```python
from build123d import *
from OCP.BRepFilletAPI import BRepFilletAPI_MakeChamfer

# Parameters (mm, degrees)
BOSS_EXTRUDE1_DEPTH                               = 38
SKETCH5_W                                         = 63
SKETCH5_H                                         = 38
BOSS_EXTRUDE2_DEPTH                               = 1.6
CHAMFER6_SIZE                                     = 0.8
CHAMFER6_SIZE2                                    = 0.738449877
CHAMFER7_SIZE                                     = 0.8
CHAMFER7_SIZE2                                    = 0.880050294
CHAMFER7_SIZE2_2                                  = 0.59857957
CSK_FOR_6_FLAT_HEAD_MACHINE_SCREW_100_D           = 4.3053
CSK_FOR_6_FLAT_HEAD_MACHINE_SCREW_100_DEPTH       = 3.6
CSK_FOR_6_FLAT_HEAD_MACHINE_SCREW_100_CSINK_D     = 7.0866
CSK_FOR_6_FLAT_HEAD_MACHINE_SCREW_100_CSINK_ANGLE = 100
FILLET1_R                                         = 10
CHAMFER10_SIZE                                    = 1.5


with BuildPart() as part:
    # Sketch1 → Boss-Extrude1 (new body)
    with BuildSketch(Plane.XY):
        Polygon((-34.595581798, 39), (-29.986555798, 39), (-32.97810591, 45.15618727), (-31.179250624, 46.030326652), (-27.76291945, 39), (-27.76291945, 37), (-32.76291945, 37), (-36, 0), (0, 0), (36, 0), (32.76291945, 37), (27.76291945, 37), (27.76291945, 39), (31.179250624, 46.030326652), (32.97810591, 45.15618727), (29.986555798, 39), (34.595581798, 39), (38.182617002, -2), (0, -2), (-38.182617002, -2), align=None)
    extrude(amount=BOSS_EXTRUDE1_DEPTH)

    # Sketch5 → Boss-Extrude2 (add)
    with BuildSketch(Plane.XZ.offset(2)):
        with Locations((0, 19)):
            Rectangle(SKETCH5_W, SKETCH5_H)
    extrude(amount=BOSS_EXTRUDE2_DEPTH)

    # Chamfer6: one chamfer whose edges measure the first distance from different faces: ONE call of the kernel's chamfer builder (chamfer() names one face for all edges)
    chamfer6_edges_1 = [part.edges().sort_by_distance(p)[0] for p in [
        (-36, 0, 19),
    ]]
    chamfer6_side_1 = [part.faces().sort_by_distance(p)[0] for p in [
        (0, 0, 19),
    ]]
    chamfer6_edges_2 = [part.edges().sort_by_distance(p)[0] for p in [
        (36, 0, 19),
    ]]
    chamfer6_side_2 = [part.faces().sort_by_distance(p)[0] for p in [
        (34.381459725, 18.5, 19),
    ]]
    chamfer6_edges_3 = [part.edges().sort_by_distance(p)[0] for p in [
        (38.182617002, -2, 19),
    ]]
    chamfer6_side_3 = [part.faces().sort_by_distance(p)[0] for p in [
        (34.841308501, -2, 19),
    ]]
    chamfer6_edges_4 = [part.edges().sort_by_distance(p)[0] for p in [
        (-38.182617002, -2, 19),
    ]]
    chamfer6_side_4 = [part.faces().sort_by_distance(p)[0] for p in [
        (-36.3890994, 18.5, 19),
    ]]
    chamfer6 = BRepFilletAPI_MakeChamfer(part.part.solid().wrapped)
    for e in chamfer6_edges_1:
        chamfer6.Add(CHAMFER6_SIZE, CHAMFER6_SIZE2, e.wrapped, chamfer6_side_1[0].wrapped)  # the first distance lies on this face
    for e in chamfer6_edges_2:
        chamfer6.Add(CHAMFER6_SIZE, CHAMFER6_SIZE2, e.wrapped, chamfer6_side_2[0].wrapped)  # the first distance lies on this face
    for e in chamfer6_edges_3:
        chamfer6.Add(CHAMFER6_SIZE, CHAMFER6_SIZE2, e.wrapped, chamfer6_side_3[0].wrapped)  # the first distance lies on this face
    for e in chamfer6_edges_4:
        chamfer6.Add(CHAMFER6_SIZE, CHAMFER6_SIZE2, e.wrapped, chamfer6_side_4[0].wrapped)  # the first distance lies on this face
    add(Compound.cast(chamfer6.Shape()), mode=Mode.REPLACE)

    # Chamfer7: one chamfer whose edges measure the first distance from different faces: ONE call of the kernel's chamfer builder (chamfer() names one face for all edges)
    chamfer7_edges_1 = [part.edges().sort_by_distance(p)[0] for p in [
        (-32.76291945, 37, 19),
    ]]
    chamfer7_side_1 = [part.faces().sort_by_distance(p)[0] for p in [
        (-34.349279651, 18.867819926, 19),
    ]]
    chamfer7_edges_2 = [part.edges().sort_by_distance(p)[0] for p in [
        (32.76291945, 37, 19),
    ]]
    chamfer7_side_2 = [part.faces().sort_by_distance(p)[0] for p in [
        (30.26291945, 37, 19),
    ]]
    chamfer7_edges_3 = [part.edges().sort_by_distance(p)[0] for p in [
        (29.986555798, 39, 19),
    ]]
    chamfer7_side_3 = [part.faces().sort_by_distance(p)[0] for p in [
        (32.291068798, 39, 19),
    ]]
    chamfer7_edges_4 = [part.edges().sort_by_distance(p)[0] for p in [
        (34.595581798, 39, 19),
    ]]
    chamfer7_side_4 = [part.faces().sort_by_distance(p)[0] for p in [
        (36.356919326, 18.867819926, 19),
    ]]
    chamfer7_edges_5 = [part.edges().sort_by_distance(p)[0] for p in [
        (-34.595581798, 39, 19),
    ]]
    chamfer7_side_5 = [part.faces().sort_by_distance(p)[0] for p in [
        (-32.291068798, 39, 19),
    ]]
    chamfer7_edges_6 = [part.edges().sort_by_distance(p)[0] for p in [
        (-29.986555798, 39, 19),
    ]]
    chamfer7_side_6 = [part.faces().sort_by_distance(p)[0] for p in [
        (-31.482330854, 42.078093635, 19),
    ]]
    chamfer7 = BRepFilletAPI_MakeChamfer(part.part.solid().wrapped)
    for e in chamfer7_edges_1:
        chamfer7.Add(CHAMFER7_SIZE, CHAMFER7_SIZE2, e.wrapped, chamfer7_side_1[0].wrapped)  # the first distance lies on this face
    for e in chamfer7_edges_2:
        chamfer7.Add(CHAMFER7_SIZE, CHAMFER7_SIZE2, e.wrapped, chamfer7_side_2[0].wrapped)  # the first distance lies on this face
    for e in chamfer7_edges_3:
        chamfer7.Add(CHAMFER7_SIZE, CHAMFER7_SIZE2_2, e.wrapped, chamfer7_side_3[0].wrapped)  # the first distance lies on this face
    for e in chamfer7_edges_4:
        chamfer7.Add(CHAMFER7_SIZE, CHAMFER7_SIZE2, e.wrapped, chamfer7_side_4[0].wrapped)  # the first distance lies on this face
    for e in chamfer7_edges_5:
        chamfer7.Add(CHAMFER7_SIZE, CHAMFER7_SIZE2, e.wrapped, chamfer7_side_5[0].wrapped)  # the first distance lies on this face
    for e in chamfer7_edges_6:
        chamfer7.Add(CHAMFER7_SIZE, CHAMFER7_SIZE2_2, e.wrapped, chamfer7_side_6[0].wrapped)  # the first distance lies on this face
    add(Compound.cast(chamfer7.Shape()), mode=Mode.REPLACE)

    # CSK for #6 Flat Head Machine Screw (100)1
    with Locations(Plane(origin=(0, 0, 0), x_dir=(1, 0, 0), z_dir=(0, 1, 0))):
        with Locations((24.3, -19), (-24.3, -19)):
            CounterSinkHole(CSK_FOR_6_FLAT_HEAD_MACHINE_SCREW_100_D / 2, CSK_FOR_6_FLAT_HEAD_MACHINE_SCREW_100_CSINK_D / 2, depth=CSK_FOR_6_FLAT_HEAD_MACHINE_SCREW_100_DEPTH, counter_sink_angle=CSK_FOR_6_FLAT_HEAD_MACHINE_SCREW_100_CSINK_ANGLE)

    # Fillet1
    fillet1_edges = [part.edges().sort_by_distance(p)[0] for p in [
        (-31.5, -2.8, 0),
        (31.5, -2.8, 0),
        (31.5, -2.8, 38),
        (-31.5, -2.8, 38),
    ]]
    fillet(fillet1_edges, radius=FILLET1_R)

    # Chamfer10
    chamfer10_edges = [part.edges().sort_by_distance(p)[0] for p in [
        (-31.5, -3.6, 19),
        (0, -3.6, 38),
        (0, -3.6, 0),
        (31.5, -3.6, 19),
        (28.571067812, -3.6, 35.071067812),
        (28.571067812, -3.6, 2.928932188),
        (-28.571067812, -3.6, 2.928932188),
        (-28.571067812, -3.6, 35.071067812),
    ]]
    chamfer(chamfer10_edges, length=CHAMFER10_SIZE)


solid = part.part
```
Model file for the job. Use its own axes, mm. A direction names the side the tool comes from. Coordinates: 2 decimals unless noted, no trailing zeros. Write each loop counter-clockwise with the first axis right and the second up, starting at its lowest first coordinate (ties: lowest second). Pieces come first, ordered by that corner, then holes. Notation, with made-up numbers: (-27.5, -4.5) - (-9.5, -4.5) arc R28 cw to (-9.5, 14.5) - close; hole circle Ø6 at (10.25, -13.75). An arc over 180 degrees is marked (long way). One line per item, written item: value. Start each with the question number.
1. Probe line 1 (Z direction, x = -24.3, y = -1.9); line 2 (X direction, y = -2.75, z = 19); line 3 (X direction, y = -1.9, z = 19). List the from-to ranges inside material, lowest first. Write a range as from..to.
2. Tool access for faces 4 (the flat face through (31.632, 42.387, 18.734)), 5 (the flat face through (-32, 39, 19)), 6 (the flat face through (-30, 37, 19)), 7 (the flat face through (29.45, 42.47, 18.73)): list every direction of +Z, -Z, +X, -X, +Y, -Y with a clear straight run to the whole face (end or side of a thin tool).
3. Mould opens along Z. For faces 1 (the flat face through (-27.763, 38, 19)), 2 (the flat face through (0.3, -2.9, 0.8)), 3 (the flat face through (-0.3, -2.9, 37.2)) say: released by +Z, released by -Z, zero draft, split by the parting line, or undercut.
4. Slice it at C-C (x = -9.5). Write the cut outline in (y, z), plus the area to 3 significant figures.
5. Flat gauge pins, fed straight in: pin 1 (0.6 mm diameter, centred on y = 38, z = 20.5, fed in from +X); pin 2 (3.5 mm diameter, centred on x = -24.3, z = 19, fed in from +Y); pin 3 (5 mm diameter, centred on y = 20.5, z = 33, fed in from -X); pin 4 (1 mm diameter, centred on y = 18.5, z = 5, fed in from +X). Where does each tip first touch, or does it go through?
6. Slice it at B-B (y = 6). Write the cut outline in (x, z), plus the area to 3 significant figures.
Answers below:
1. line 1: z = 0..16.85, 21.15..38
1. line 2: x = -30.85..-26.45, -22.15..22.15, 26.45..30.85
1. line 3: x = -37.53..-26.45, -22.15..22.15, 26.45..37.48
2. face 4: +Z, -Z, +X
2. face 5: +Z, -Z, -X
2. face 6: +Z, -Z
2. face 7: +Z, -Z, +Y
3. face 1: zero draft
3. face 2: released by -Z
3. face 3: released by +Z
4. outline: (-3.6, 1.5) - (-2.1, 0) - (0, 0) - (0, 38) - (-2.1, 38) - (-3.6, 36.5) - close
4. area: 135 mm^2
5. pin 1: stops at x = 34.71
5. pin 2: passes through
5. pin 3: stops at x = -36.43
5. pin 4: stops at x = 36.43
6. outline: (-37.48, 0) - (-35.48, 0) - (-35.48, 38) - (-37.48, 38) - close; (35.48, 0) - (37.48, 0) - (37.48, 38) - (35.48, 38) - close
6. area: 153 mm^2
